from build123d import *

# Parameters (mm, degrees)
BODYSCH_R       = 14.2875
BODY_DEPTH      = 47.625
FLOWSCH_R       = 9.128125
FLOW_DEPTH      = 20.3454
FLOWSMALLSCH_R  = 7.62
FLOWSMALL_DEPTH = 43.409911534


# Read off the part's stored shape, not the designer's step: Flow30deg
with BuildPart() as part:
    # BodySch → Body (new body)
    with BuildSketch(Plane.XY):
        Circle(BODYSCH_R)
    extrude(amount=BODY_DEPTH)

    # FlowSch → Flow (cut)
    with BuildSketch(Plane.XY.offset(47.625)):
        Circle(FLOWSCH_R)
    extrude(amount=-FLOW_DEPTH, mode=Mode.SUBTRACT)

    # ThreadSch → Thread (revolve, cut)
    with BuildSketch(Plane(origin=(0, 0, 0), x_dir=(0, 0, -1), z_dir=(1, 0, 0)), mode=Mode.PRIVATE) as thread_sk:
        Polygon((-34.0614, 0), (-34.0614, 10.24569605), (-47.625, 10.668), (-47.625, 0), align=None)
    revolve(thread_sk.sketch.rotate(Axis((0, 0, 0), (0, 0, 1)), 90), axis=Axis((0, 0, 0), (0, 0, 1)), mode=Mode.SUBTRACT)

    # ThreadSmallSke → ThreadSmall (revolve, cut)
    with BuildSketch(Plane(origin=(0, 0, 0), x_dir=(0, 0, -1), z_dir=(1, 0, 0)), mode=Mode.PRIVATE) as threadsmall_sk:
        Polygon((0, 0), (0, 8.5725), (-10.3378, 8.250631633), (-10.3378, 0), (-0.549620086, 0), align=None)
    revolve(threadsmall_sk.sketch.rotate(Axis((0, 0, 0), (0, 0, 1)), 90), axis=Axis((0, 0, 0), (0, 0, 1)), mode=Mode.SUBTRACT)

    # Flow30deg outline → Flow30deg (revolve, cut)
    with BuildSketch(Plane.XZ):
        Polygon((0, 27.2796), (0, 11.469223722), (9.128125, 27.2796), align=None)
    revolve(axis=Axis((0, 0, 0), (0, 0, 1)), mode=Mode.SUBTRACT)

    # FlowSmallSch → FlowSmall (cut, through all)
    with BuildSketch(Plane(origin=(0, 0, 10.3378), x_dir=(-1, 0, 0), z_dir=(0, 0, -1))):
        Circle(FLOWSMALLSCH_R)
    extrude(amount=-FLOWSMALL_DEPTH, mode=Mode.SUBTRACT)


solid = part.part
Read the model definition and answer for the solid it produces. Units are mm, in the model's axes. A direction names the side the tool comes from. Coordinates: 2 decimals unless noted, no trailing zeros. Loops run counter-clockwise (first coordinate to the right, second up) from the corner with the lowest first, then second, coordinate; pieces in that order, holes last. Notation, with made-up numbers: (79, -29) -> (114, -29) arc R37 ccw to (114, 7) -> close; hole circle Ø2 at (17.25, -4). An arc over 180 degrees is marked (long way). Write item = value, one per line. Start each with the question number.
1) The part is cut by section D-D, the plane y = 12. Determine the outline of the cut face in (x, z) (3 decimals), plus the area to 3 significant figures.
2) The mould has two halves that part along X. Classify faces 1 (the face through (-14.274, 0.628, 23.479)), 2 (the face through (-9.2, 1.5, 34.061)), 3 (the face through (0, -9, 0)): pulls with the +X half, pulls with the -X half, needs draft (parallel to the pull), parting line crosses it, or undercut.
3) The part is cut by section A-A, the plane y = 0. Determine the outline of the cut face in (x, z) (1 decimal), plus the area to 3 significant figures.
4) Given P1, Ø8, axis at x = 3, y = 6, coming from the +Z side (3 decimals); P2, Ø10, axis at x = 2, y = 4, coming from the +Z side; P3, Ø3, axis at y = -8.5, z = 12.5, coming from the +X side; P4, Ø11, axis at x = 0, y = 0, coming from the -Z side, each flat-ended and moving along its own axis, determine where each tip first touches the part or whether it passes through.
5) For faces 4 (the face through (2.27, 10.21, 40.94)), 5 (the face through (-5.5, 5.5, 10.338)), 6 (the face through (-11, -1, 47.625)), determine the directions among +Z, -Z, +X, -X, +Y, -Y from which every point of the face is accessible in a straight line to the end or side of a thin tool.
6) The part is cut by section C-C, the plane z = 39. Determine the outline of the cut face in (x, y) (1 decimal), plus the area to 3 significant figures.
7) Find the intervals of material crossed by L1, parallel to Y at x = 0, z = 15.75; L2, parallel to Y at x = 0, z = 31; L3, parallel to Y at x = 11, z = 40, in increasing order. Write a range as from..to.
Result:
q1.outline = (-7.755, 0) -> (7.755, 0) -> (7.755, 47.625) -> (-7.755, 47.625) -> close
q1.area = 739 mm²
q2.face_1 = parting line crosses it
q2.face_2 = undercut
q2.face_3 = needs draft
q3.outline = (-14.3, 0) -> (-8.6, 0) -> (-8.3, 10.3) -> (-7.6, 10.3) -> (-7.6, 24.7) -> (-9.1, 27.3) -> (-9.1, 34.1) -> (-10.2, 34.1) -> (-10.7, 47.6) -> (-14.3, 47.6) -> close; (7.6, 10.3) -> (8.3, 10.3) -> (8.6, 0) -> (14.3, 0) -> (14.3, 47.6) -> (10.7, 47.6) -> (10.2, 34.1) -> (9.1, 34.1) -> (9.1, 27.3) -> (7.6, 24.7) -> close
q3.area = 517 mm²
q4.P1 = 47.625
q4.P2 = 34.06
q4.P3 = 12.46
q4.P4 = through
q5.face_4 = +Z
q5.face_5 = -Z
q5.face_6 = +Z, +X, -X, +Y, -Y
q6.outline = circle Ø28.6 at (0, 0); hole circle Ø20.8 at (0, 0)
q6.area = 302 mm²
q7.L1 = -14.29..-7.62, 7.62..14.29
q7.L2 = -14.29..-9.13, 9.13..14.29
q7.L3 = -9.12..9.12
